```python
from build123d import *

# Parameters (mm, degrees)
SKETCH_1_W             = 56
SKETCH_1_H             = 50
EXTRUDE_1_DEPTH        = 72
SKETCH_2_W             = 52
SKETCH_2_H             = 40
CUT_EXTRUDE_1_DEPTH    = 105.019228992
HOLE_WIZARD_M3_1_D     = 2.5
HOLE_WIZARD_M3_1_DEPTH = 7.5
HOLE_WIZARD_M3_1_TIP   = 0.751075774
CUT_EXTRUDE_2_DEPTH    = 92.323600455


with BuildPart() as part:
    # 草图1 → 凸台-拉伸1 (new body)
    with BuildSketch(Plane.XY):
        with Locations((28, 25)):
            Rectangle(SKETCH_1_W, SKETCH_1_H)
    extrude(amount=EXTRUDE_1_DEPTH)

    # 草图2 → 切除-拉伸1 (cut, through all)
    with BuildSketch(Plane(origin=(56, 0, 0), x_dir=(0, 0, -1), z_dir=(1, 0, 0))):
        with Locations((-46, 20)):
            Rectangle(SKETCH_2_W, SKETCH_2_H)
    extrude(amount=-CUT_EXTRUDE_1_DEPTH, mode=Mode.SUBTRACT)

    # M3 螺纹孔1
    with Locations(Plane(origin=(0, 50, 0), x_dir=(-1, 0, 0), z_dir=(0, 1, 0))):
        with Locations((-28, 67.25), (-28, 33.25), (-18, 50.25), (-38, 50.25)):
            Hole(HOLE_WIZARD_M3_1_D / 2, depth=HOLE_WIZARD_M3_1_DEPTH)
            with Locations((0, 0, -(HOLE_WIZARD_M3_1_DEPTH + HOLE_WIZARD_M3_1_TIP / 2))):  # 118° drill point
                Cone(0, HOLE_WIZARD_M3_1_D / 2, HOLE_WIZARD_M3_1_TIP, mode=Mode.SUBTRACT)

    # 草图5 → 切除-拉伸2 (cut, through all)
    with BuildSketch(Plane.XY.offset(20)):
        with BuildLine():
            Line((10, 32.7), (18, 32.7))
            ThreePointArc((18, 32.7), (20.7, 30), (18, 27.3))
            Line((18, 27.3), (10, 27.3))
            ThreePointArc((10, 27.3), (7.3, 30), (10, 32.7))
        make_face()
        with BuildLine():
            Line((46, 32.7), (38, 32.7))
            ThreePointArc((38, 32.7), (35.3, 30), (38, 27.3))
            Line((38, 27.3), (46, 27.3))
            ThreePointArc((46, 27.3), (48.7, 30), (46, 32.7))
        make_face()
        with BuildLine():
            Line((10, 7.3), (18, 7.3))
            ThreePointArc((18, 7.3), (20.7, 10), (18, 12.7))
            Line((18, 12.7), (10, 12.7))
            ThreePointArc((10, 12.7), (7.3, 10), (10, 7.3))
        make_face()
        with BuildLine():
            Line((46, 7.3), (38, 7.3))
            ThreePointArc((38, 7.3), (35.3, 10), (38, 12.7))
            Line((38, 12.7), (46, 12.7))
            ThreePointArc((46, 12.7), (48.7, 10), (46, 7.3))
        make_face()
    extrude(amount=-CUT_EXTRUDE_2_DEPTH, mode=Mode.SUBTRACT)


solid = part.part
```
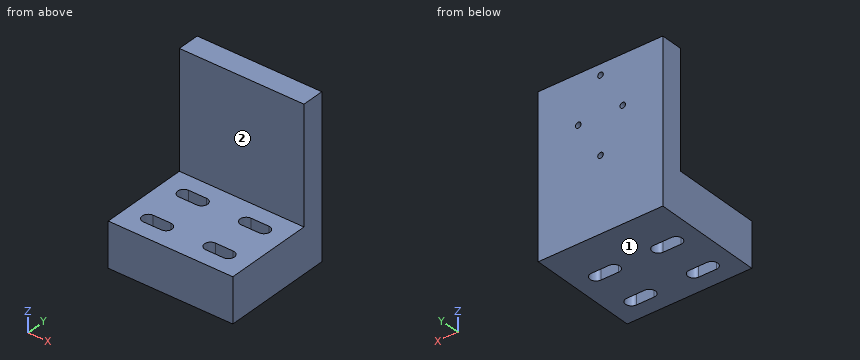
Work out the finished part from the listing and answer in its coordinate system (mm). Face numbers are marked on the shaded views. A direction names the side the tool comes from. Round coordinates to 2 decimals unless told otherwise and drop trailing zeros. Order: outer loops, then holes, each group sorted by start corner. A loop starts at its lowest first (then second) coordinate and runs counter-clockwise, first axis right, second up.
Q1. Find the intervals of material crossed by line 1 along Z through (x, y) = (28, 47.75); line 2 along Z through (x, y) = (38, 45.25); line 3 along Y through (x, z) = (17, 3.5), in increasing order.
Solution:
line 1: z = 0 to 32, 34.5 to 66, 68.5 to 72
line 2: z = 0 to 49, 51.5 to 72
line 3: y = 0 to 7.3, 12.7 to 27.3, 32.7 to 50
Q2. Given pin 1 Ø9 at (x, z) = (16, 7.5) entering from -Y; pin 2 Ø2 at (x, z) = (28, 67.25) entering from -Y, each flat-ended and moving along its own axis, determine where each tip first touches the part or whether it passes through.
Solution:
pin 1: stops at y = 0
pin 2: stops at y = 40
Q3. A cutting plane is placed at B-B, the plane z = 9. Determine the outline of the cut face in (x, y), then the cut area to 3 significant figures.
Solution:
outline: (0, 0) - (56, 0) - (56, 50) - (0, 50) - close; hole (10, 7.3) - (18, 7.3) arc R2.7 ccw to (18, 12.7) - (10, 12.7) arc R2.7 ccw to start; hole (10, 27.3) - (18, 27.3) arc R2.7 ccw to (18, 32.7) - (10, 32.7) arc R2.7 ccw to start; hole (38, 7.3) - (46, 7.3) arc R2.7 ccw to (46, 12.7) - (38, 12.7) arc R2.7 ccw to start; hole (38, 27.3) - (46, 27.3) arc R2.7 ccw to (46, 32.7) - (38, 32.7) arc R2.7 ccw to start
area: 2,540 mm2
Q4. A tool of negligible diameter and unlimited length cuts with its end or side. For the marked faces 1 and 2, from which of +Z, -Z, +X, -X, +Y, -Y can it reach the whole face along a straight path? Write none if from no direction.
Solution:
face 1: -Z, +X, -X, +Y, -Y
face 2: +Z, +X, -X, -Y
Q5. A cutting plane is placed at A-A, the plane x = 12.5. Determine the outline of the cut face in (y, z), then the cut area to 3 significant figures.
Solution:
outline: (0, 0) - (7.3, 0) - (7.3, 20) - (0, 20) - close; (12.7, 0) - (27.3, 0) - (27.3, 20) - (12.7, 20) - close; (32.7, 0) - (50, 0) - (50, 72) - (40, 72) - (40, 20) - (32.7, 20) - close
area: 1,300 mm2
Q6. A cutting plane is placed at D-D, the plane z = 40. Determine the outline of the cut face in (x, y).
Solution:
outline: (0, 40) - (56, 40) - (56, 50) - (0, 50) - close
Q7. A cutting plane is placed at C-C, the plane x = 24. Determine the outline of the cut face in (y, z).
Solution:
outline: (0, 0) - (50, 0) - (50, 72) - (40, 72) - (40, 20) - (0, 20) - close
